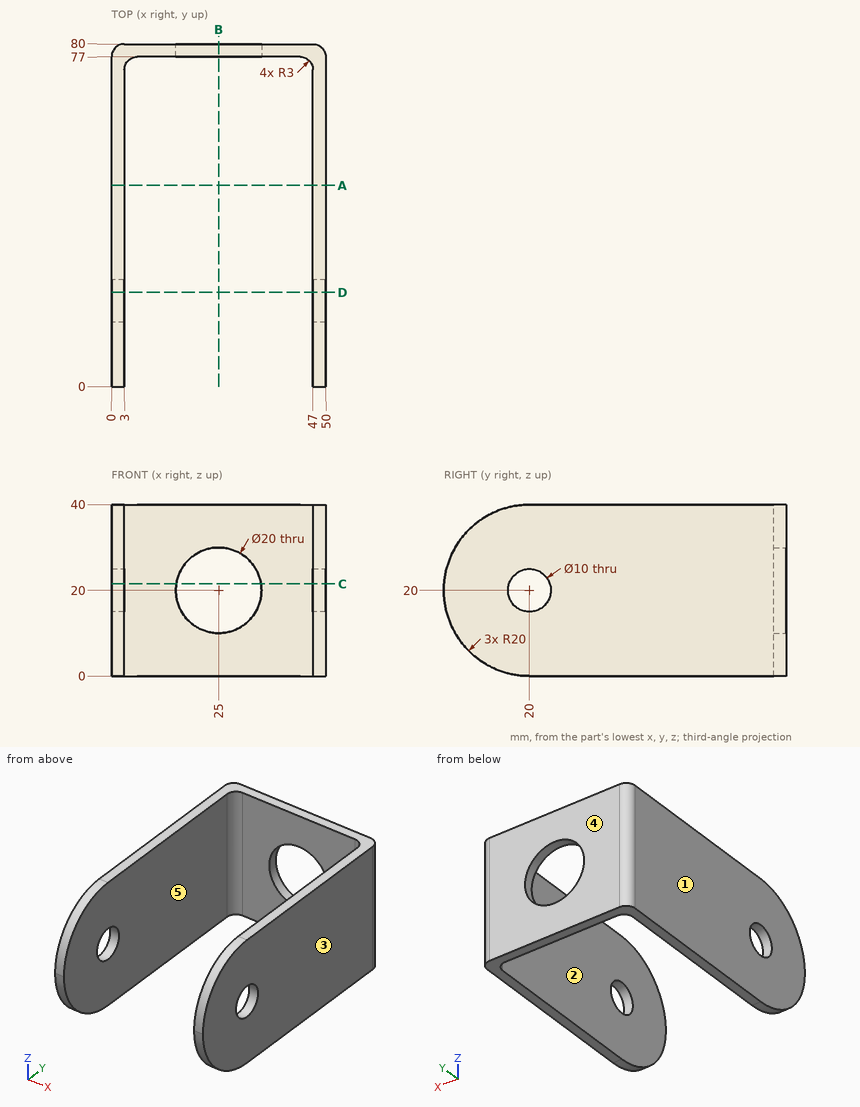
Drawing for the job (mm, zero at the part's lowest x, y, z). A direction names the side the tool comes from. Give positions to 0.01 mm unless a question says otherwise; leave off trailing zeros. Order: outer loops, then holes, each group sorted by start corner. A loop starts at its lowest first (then second) coordinate and runs counter-clockwise, first axis right, second up. Notation, with made-up numbers: (40.25, 86) -> (73.25, 86) arc R15 ccw to (73.25, 115) -> close; hole circle Ø11 at (-5, 20.5). An arc over 180 degrees is marked (long way). Use one line per item in the form item = value.
(1) Drill centre lines: line 1 (Z direction, x = 25, y = 78.7); line 2 (X direction, y = 57, z = 9); line 3 (Y direction, x = 48, z = 20). Where is each one in solid material? Low to high. Write a range as from..to.
Solution:
line_1 = 0..10, 30..40
line_2 = 0..3, 47..50
line_3 = 0..15, 25..79.83
(2) Tool access for the marked faces 1 and 2: list every direction of +Z, -Z, +X, -X, +Y, -Y with a clear straight run to the whole face (end or side of a thin tool).
Solution:
face_1 = +Z, -Z, -X, +Y, -Y
face_2 = +Z, -Z, -Y
(3) Saw through at C-C (z = 21.5). Write the cut outline in (x, y).
Solution:
outline = (0, 0.06) -> (3, 0.06) -> (3, 15.23) -> (0, 15.23) -> close; (0, 24.77) -> (3, 24.77) -> (3, 74) arc R3 cw to (6, 77) -> (15.11, 77) -> (15.11, 80) -> (3, 80) arc R3 ccw to (0, 77) -> close; (34.89, 77) -> (44, 77) arc R3 cw to (47, 74) -> (47, 24.77) -> (50, 24.77) -> (50, 77) arc R3 ccw to (47, 80) -> (34.89, 80) -> close; (47, 0.06) -> (50, 0.06) -> (50, 15.23) -> (47, 15.23) -> close
(4) Saw through at B-B (x = 25). Write the cut outline in (y, z).
Solution:
outline = (77, 0) -> (80, 0) -> (80, 10) -> (77, 10) -> close; (77, 30) -> (80, 30) -> (80, 40) -> (77, 40) -> close
(5) Flat gauge pins, fed straight in: P1, Ø5, axis at x = 38.5, z = 11, coming from the -Y side; P2, Ø2, axis at y = 18.5, z = 12.5, coming from the -X side; P3, Ø6, axis at y = 20, z = 20, coming from the -X side. Where does each tip first touch, or does it go through?
Solution:
P1 = 77
P2 = 0
P3 = through
(6) Saw through at D-D (y = 22). Write the cut outline in (x, z), then the cut area to 3 significant figures.
Solution:
outline = (0, 0) -> (3, 0) -> (3, 15.42) -> (0, 15.42) -> close; (0, 24.58) -> (3, 24.58) -> (3, 40) -> (0, 40) -> close; (47, 0) -> (50, 0) -> (50, 15.42) -> (47, 15.42) -> close; (47, 24.58) -> (50, 24.58) -> (50, 40) -> (47, 40) -> close
area = 185 mm²
(7) Saw through at A-A (y = 47). Write the cut outline in (x, z).
Solution:
outline = (0, 0) -> (3, 0) -> (3, 40) -> (0, 40) -> close; (47, 0) -> (50, 0) -> (50, 40) -> (47, 40) -> close
(8) Pull direction X, two halves, no side cores. Call the marked faces 3, 4 and 5: +X half, -X half, draft (parallel to the pull), parting line (faces both ways), or undercut.
Solution:
face_3 = +X half
face_4 = draft
face_5 = undercut
